```python
from build123d import *

# Parameters (mm, degrees)
BOSS_EXTRUDE1_DEPTH = 19.05
BOSS_EXTRUDE2_DEPTH = 19.05
CHAMFER1_SIZE       = 12.7
CHAMFER1_SIZE2      = 11.325028866
SKETCH12_W          = 31.75
SKETCH12_H          = 76.2
CUT_EXTRUDE1_DEPTH  = 367.085742005
FILLET1_R           = 12.7


# Read off the part's stored shape, not the designer's step: Hole3, Hole4
with BuildPart() as part:
    # Sketch2 → Boss-Extrude1 (new body)
    with BuildSketch(Plane(origin=(-113.788766336, 0, 0), x_dir=(0, 0, -1), z_dir=(1, 0, 0))):
        with BuildLine():
            Line((0, 20.824633003), (-83.828599938, 40.306941911))
            Line((-83.828599938, 40.306941911), (-93.196193981, 0))
            Line((-93.196193981, 0), (-63.5, 0))
            ThreePointArc((-63.5, 0), (-58.07993597, 2.24506403), (-60.325, -3.175))
            Line((-60.325, -3.175), (-60.325, -298.45))
            Line((-60.325, -298.45), (0, -298.45))
            Line((0, -298.45), (0, 20.824633003))
        make_face()
    extrude(amount=BOSS_EXTRUDE1_DEPTH)

    # Sketch3 → Boss-Extrude2 (add, through all)
    with BuildSketch(Plane.ZY.offset(113.788766336)):
        Polygon((83.828599938, 40.306941911), (201.08567571, 67.558244849), (214.022912031, 11.891823944), (93.196193981, 0), align=None)
    extrude(amount=-BOSS_EXTRUDE2_DEPTH)

    # Chamfer1
    chamfer1_edges = [part.edges().sort_by_distance(p)[0] for p in [
        (-104.263766336, 11.891823944, 214.022912031),
    ]]
    chamfer1_side = [part.faces().sort_by_distance(p)[0] for p in [
        (-104.263766336, 39.725034397, 207.554293871),
    ]]
    chamfer(chamfer1_edges, length=CHAMFER1_SIZE, length2=CHAMFER1_SIZE2, reference=chamfer1_side[0])

    # Hole3 outline → Hole3 (revolve, cut)
    with BuildSketch(Plane(origin=(-104.263766336, 5.379568105, 23.147239101), x_dir=(1, 0, 0), z_dir=(0, 0.22637333895091205, 0.9740406107612842))):
        Polygon((0, 0.280172016), (1.5875, 1.234038249), (1.5875, 20.284038249), (0, 20.284038249), align=None)
    revolve(axis=Axis((-104.263766336, 5.379568105, 23.147239101), (0, 0.9740406107612842, -0.22637333895091205)), mode=Mode.SUBTRACT)

    # Hole3 2 outline → Hole3 2 (revolve, cut)
    with BuildSketch(Plane(origin=(-104.263766336, 24.433961921, 105.134603321), x_dir=(1, 0, 0), z_dir=(0, 0.22637333895091205, 0.9740406107612842))):
        Polygon((0, 0.280172016), (1.5875, 1.234038249), (1.5875, 20.284038249), (0, 20.284038249), align=None)
    revolve(axis=Axis((-104.263766336, 24.433961921, 105.134603321), (0, 0.9740406107612842, -0.22637333895091205)), mode=Mode.SUBTRACT)

    # Hole3 3 outline → Hole3 3 (revolve, cut)
    with BuildSketch(Plane(origin=(-104.263766336, 43.488355737, 187.121967541), x_dir=(1, 0, 0), z_dir=(0, 0.22637333895091205, 0.9740406107612842))):
        Polygon((0, 0.280172016), (1.5875, 1.234038249), (1.5875, 20.284038249), (0, 20.284038249), align=None)
    revolve(axis=Axis((-104.263766336, 43.488355737, 187.121967541), (0, 0.9740406107612842, -0.22637333895091205)), mode=Mode.SUBTRACT)

    # Hole4 outline → Hole4 (revolve, cut)
    with BuildSketch(Plane(origin=(-104.263766336, -279.4, 0), x_dir=(1, 0, 0), z_dir=(0, -1, 0))):
        Polygon((1.5875, 0), (1.5875, 12.7), (0, 13.653866233), (0, 0), align=None)
    revolve(axis=Axis((-104.263766336, -279.4, 0), (0, 0, 1)), mode=Mode.SUBTRACT)

    # Hole4 2 outline → Hole4 2 (revolve, cut)
    with BuildSketch(Plane(origin=(-104.263766336, -149.225, 0), x_dir=(1, 0, 0), z_dir=(0, -1, 0))):
        Polygon((1.5875, 0), (1.5875, 12.7), (0, 13.653866233), (0, 0), align=None)
    revolve(axis=Axis((-104.263766336, -149.225, 0), (0, 0, 1)), mode=Mode.SUBTRACT)

    # Hole4 3 outline → Hole4 3 (revolve, cut)
    with BuildSketch(Plane(origin=(-104.263766336, -19.05, 0), x_dir=(1, 0, 0), z_dir=(0, -1, 0))):
        Polygon((1.5875, 0), (1.5875, 12.7), (0, 13.653866233), (0, 0), align=None)
    revolve(axis=Axis((-104.263766336, -19.05, 0), (0, 0, 1)), mode=Mode.SUBTRACT)

    # Sketch12 → Cut-Extrude1 (cut, through all)
    with BuildSketch(Plane(origin=(-94.738766336, 0, 0), x_dir=(0, 0, -1), z_dir=(1, 0, 0))):
        with Locations((-36.5125, -142.875)):
            Rectangle(SKETCH12_W, SKETCH12_H)
    extrude(amount=-CUT_EXTRUDE1_DEPTH, mode=Mode.SUBTRACT)

    # Fillet1
    fillet1_edges = [part.edges().sort_by_distance(p)[0] for p in [
        (-104.263766336, -104.775, 20.6375),
        (-104.263766336, -180.975, 20.6375),
        (-104.263766336, -180.975, 52.3875),
        (-104.263766336, -104.775, 52.3875),
    ]]
    fillet(fillet1_edges, radius=FILLET1_R)


solid = part.part
```
Can you work these out from the model? Positions are in its coordinate system, mm. A direction names the side the tool comes from. Round coordinates to 2 decimals unless told otherwise and drop trailing zeros. Loops run counter-clockwise (first coordinate to the right, second up) from the corner with the lowest first, then second, coordinate; pieces in that order, holes last. Notation, with made-up numbers: M 44,-3 L 60,-3 A18 cw 60,22 Z; hole C -28.5,-17 d11. An arc over 180 degrees is marked long. Write item = value, one per line. Start each with the question number.
(1) I need wall thicknesses on line 1 along Z through (x, y) = (-97.25, -161) (1 decimal); line 2 along Z through (x, y) = (-97.25, -282.5) (3 decimals); line 3 along Y through (x, z) = (-98.5, 42). Which ranges of each line are inside material? Lowest first, please.
(2) Suppose I cut it at B-B on y = -29. Write out the boundary of the cut face in (x, z) (3 decimals).
(3) Suppose I cut it at A-A on y = -158.5. Write out the boundary of the cut face in (x, z) (1 decimal), plus the area to 3 significant figures.
(4) If we mould it in two halves opening along Z, with no side actions, what happens to faces 1 (the face through (-104.397, -108.594, 24.259)), 2 (the face through (-94.739, -72, 60)), 3 (the face through (-104.397, 5.467, 148.741))? For each: released by +Z, released by -Z, zero draft, split by the parting line, or undercut.
(5) Which directions (+Z, -Z, +X, -X, +Y, -Y) give clear straight access to the entire face, cutting with the end or side of a thin tool? Please do faces 4 (the face through (-104, -104.775, 37)), 5 (the face through (-104, -149, 60.325)), 6 (the face through (-113.789, -72, 60)).
(6) I'm going to push flat-ended pins straight in: P1, Ø3, axis at x = -104.26, y = -279.4, coming from the -Z side; P2, Ø4, axis at y = 0, z = 60.325, coming from the -X side; P3, Ø9.5, axis at x = -105, z = 82.5, coming from the -Y side; P4, Ø5.5, axis at x = -106.5, y = -135, coming from the +Z side (3 decimals). Where does each tip first touch, or does it pass through?
Answer block:
q1.line_1 = 0 to 20.6, 52.4 to 60.3
q1.line_2 = 0 to 60.325
q1.line_3 = -298.45 to -180.76, -104.99 to 30.59
q2.outline = M -113.789,0 L -94.739,0 L -94.739,60.325 L -113.789,60.325 Z
q3.outline = M -113.8,0 L -94.7,0 L -94.7,20.6 L -113.8,20.6 Z; M -113.8,52.4 L -94.7,52.4 L -94.7,60.3 L -113.8,60.3 Z
q3.area = 544 mm²
q4.face_1 = undercut
q4.face_2 = zero draft
q4.face_3 = released by +Z
q5.face_4 = +X, -X
q5.face_5 = +Z, +X, -X, -Y
q5.face_6 = +Z, -Z, -X, +Y, -Y
q6.P1 = 12.75
q6.P2 = through
q6.P3 = 0
q6.P4 = 60.325
